Verification items for this drawing (mm, ordinates from the low corner). A direction names the side the tool comes from. Round coordinates to 2 decimals unless told otherwise and drop trailing zeros. Loops run counter-clockwise (first coordinate to the right, second up) from the corner with the lowest first, then second, coordinate; pieces in that order, holes last. Notation, with made-up numbers: M -8,0.5 L 5,0.5 A29 ccw 5,32.5 Z; hole C 41.25,39.5 d3. An arc over 180 degrees is marked long. One line per item, written item: value.
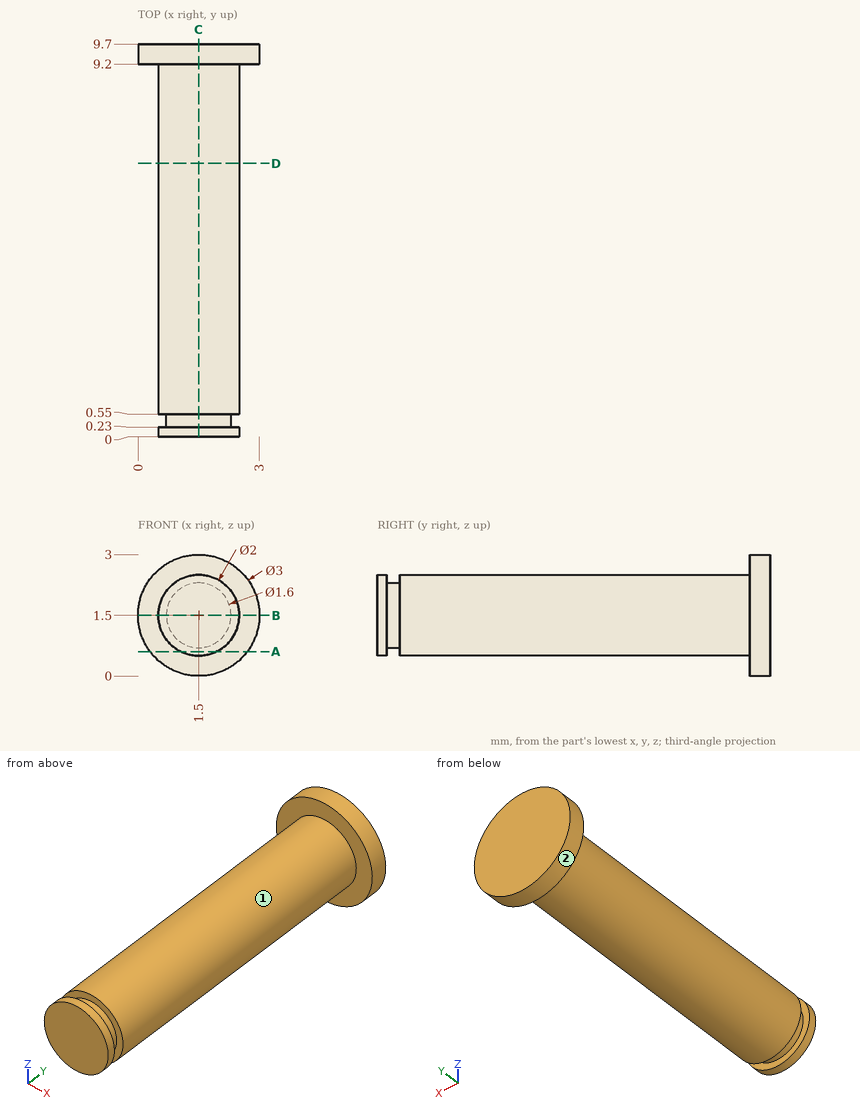
(1) Tool access check on the marked faces 1 and 2. Record the directions out of +Z, -Z, +X, -X, +Y, -Y that give a thin tool (end or side, any length) a straight path to the whole face; none if there is none.
Completed:
face 1: -Y
face 2: +Y, -Y
(2) Sectioned sample at C-C on x = 1.5. Enter the section's corners in (y, z), and give its area (3 significant figures).
Completed:
outline: M 0,0.5 L 0.23,0.5 L 0.23,0.7 L 0.55,0.7 L 0.55,0.5 L 9.2,0.5 L 9.2,0 L 9.7,0 L 9.7,3 L 9.2,3 L 9.2,2.5 L 0.55,2.5 L 0.55,2.3 L 0.23,2.3 L 0.23,2.5 L 0,2.5 Z
area: 19.8 mm^2
(3) Thickness scan on L1, parallel to Y at x = 0.75, z = 1.1; L2, parallel to Y at x = 2.6, z = 1.7; L3, parallel to Z at x = 0.9, y = 1.75. Record the ranges inside material, lowest first. Write a range as from..to.
Completed:
L1: y = 0..0.23, 0.55..9.7
L2: y = 9.2..9.7
L3: z = 0.7..2.3
(4) Sectioned sample at A-A on z = 0.6. Enter the section's corners in (x, y), and give its area (3 significant figures).
Completed:
outline: M 0.3,9.2 L 1.06,9.2 L 1.06,0.55 L 1.94,0.55 L 1.94,9.2 L 2.7,9.2 L 2.7,9.7 L 0.3,9.7 Z; M 1.06,0 L 1.94,0 L 1.94,0.23 L 1.06,0.23 Z
area: 8.94 mm^2
(5) Sectioned sample at D-D on y = 6.75. Enter the section's corners in (x, z), and give its area (3 significant figures).
Completed:
outline: C 1.5,1.5 d2
area: 3.14 mm^2
(6) Depth check by flat-ended pin: pin 1 Ø0.6 at (x, z) = (1.5, 2) entering from -Y. Enter the tip coordinate at first touch or a pass-through.
Completed:
pin 1: stops at y = 0
(7) Sectioned sample at B-B on z = 1.5. Enter the section's corners in (x, y), and give its area (3 significant figures).
Completed:
outline: M 0,9.2 L 0.5,9.2 L 0.5,0.55 L 0.7,0.55 L 0.7,0.23 L 0.5,0.23 L 0.5,0 L 2.5,0 L 2.5,0.23 L 2.3,0.23 L 2.3,0.55 L 2.5,0.55 L 2.5,9.2 L 3,9.2 L 3,9.7 L 0,9.7 Z
area: 19.8 mm^2
